Design review of the part built by this model. Coordinates are the model's own, in mm. Face numbers are marked on the shaded views. A direction names the side the tool comes from. Round coordinates to 2 decimals unless told otherwise and drop trailing zeros. Loops run counter-clockwise (first coordinate to the right, second up) from the corner with the lowest first, then second, coordinate; pieces in that order, holes last. Notation, with made-up numbers: (-10, -37.75) -> (0, -37.75) arc R17 ccw to (0, -17.75) -> close; hole circle Ø11 at (83.25, 54.25). An arc over 180 degrees is marked (long way). Answer as CSV lines item,"result". Start each with the question number.
(1) To check wall thickness, follow line 1 (Z direction, x = 9.15, y = 4.75); line 2 (Y direction, x = 10.5, z = 3); line 3 (Z direction, x = 10, y = 4.25). State the ranges of each line that lie inside material, in increasing order. Write a range as from..to.
(2) For P1, Ø1, axis at x = 11, z = -2, coming from the +Y side; P2, Ø3, axis at y = 0, z = 0, coming from the +X side, all flat-tipped, find the tip position at first contact; note any pin that passes through.
(3) Draft analysis for pull direction Z (two halves, no side actions). For the marked faces 1 and 2, state which applies: +Z half, -Z half, draft (parallel to the pull), parting line (faces both ways), or undercut.
(4) Take a section at A-A, the plane z = 0. Write out the cut boundary in (x, y), and give its area (3 significant figures).
(5) Take a section at C-C, the plane z = 2.75. Write out the cut boundary in (x, y), and give its area (3 significant figures).
(6) Machinability: for the marked faces 3 and 4, which of the approach directions +Z, -Z, +X, -X, +Y, -Y give a long, thin tool a straight path to every point of the face, cutting with its end or side? Answer none if there is none.
from build123d import *

# Parameters (mm, degrees)
BASPROSKE_W           = 12
BASPROSKE_H           = 5.6
TOOTHCUT_DEPTH        = 15.377760604
TEETHCUTS_COUNT       = 12
TEETHCUTS_ANGLE       = 330
BORSKE_R              = 2
BORE_DEPTH            = 50.0000508
CROQUIS1_W            = 12.415647279
CROQUIS1_H            = 11.755240509
CORTAR_EXTRUIR1_DEPTH = 9


with BuildPart() as part:
    # BasProSke → Base-Revolve (revolve)
    with BuildSketch(Plane(origin=(0, 0, 0), x_dir=(1, 0, 0), z_dir=(0, 1, 0)), mode=Mode.PRIVATE) as base_revolve_sk:
        with Locations((6, 2.8)):
            Rectangle(BASPROSKE_W, BASPROSKE_H)
    revolve(base_revolve_sk.sketch.rotate(Axis((-10, 0, 0), (1, 0, 0)), 180), axis=Axis((-10, 0, 0), (1, 0, 0)))

    # TooCutSke → ToothCut (cut, through all)
    with BuildSketch(Plane(origin=(0, 0, 0), x_dir=(0, 0, -1), z_dir=(1, 0, 0))):
        with BuildLine():
            ThreePointArc((0.449218713, 3.77234722), (0, 3.799), (-0.449218713, 3.77234722))
            ThreePointArc((-0.449218713, 3.77234722), (-0.670924606, 4.73673149), (-1.343429094, 5.462629717))
            ThreePointArc((-1.343429094, 5.462629717), (0, 5.6254), (1.343429094, 5.462629717))
            ThreePointArc((1.343429094, 5.462629717), (0.670924606, 4.73673149), (0.449218713, 3.77234722))
        make_face()
    toothcut = extrude(amount=TOOTHCUT_DEPTH, mode=Mode.SUBTRACT)

    # TeethCuts: ToothCut ×12 about axis
    teethcuts_axis = Axis((-10, 0, 0), (1, 0, 0))
    for i in range(1, TEETHCUTS_COUNT):
        add(toothcut.rotate(teethcuts_axis, i * TEETHCUTS_ANGLE / (TEETHCUTS_COUNT - 1)), mode=Mode.SUBTRACT)

    # BorSke → Bore (cut, symmetric)
    with BuildSketch(Plane(origin=(0, 0, 0), x_dir=(0, 0, -1), z_dir=(1, 0, 0))):
        with Locations(Location((0, 0, 0), (0, 0, 180))):
            Circle(BORSKE_R)
    extrude(amount=BORE_DEPTH, both=True, mode=Mode.SUBTRACT)

    # Croquis1 → Cortar-Extruir1 (cut)
    with BuildSketch(Plane.ZY):
        with Locations((0.242149149, 0.154094914)):
            Rectangle(CROQUIS1_W, CROQUIS1_H)
    extrude(amount=-CORTAR_EXTRUIR1_DEPTH, mode=Mode.SUBTRACT)


solid = part.part
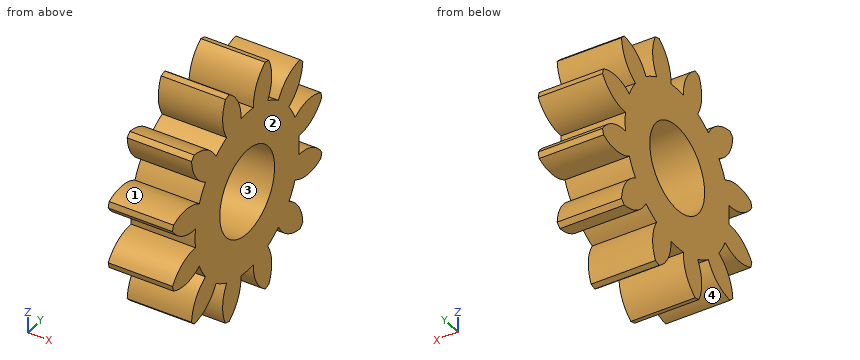
The answers:
1,line 1,"-1.77..-0.68, 0.68..1.77"
1,line 2,"-3.8..3.8"
1,line 3,"-1.77..-0.49, 0.49..1.77"
2,P1,"y = 5.4"
2,P2,"through"
3,face 1,"undercut"
3,face 2,"draft"
4,outline,"(9, -3.8) -> (12, -3.8) -> (12, -2) -> (9, -2) -> close; (9, 2) -> (12, 2) -> (12, 3.8) -> (9, 3.8) -> close"
4,area,"10.8 mm²"
5,outline,"(9, -3.62) -> (12, -3.62) -> (12, 3.62) -> (9, 3.62) -> close"
5,area,"21.7 mm²"
6,face 3,"+X, -X"
6,face 4,"-Z, +X, -X"
